from build123d import *

# Parameters (mm, degrees)
SKETCH1_R               = 6.25
BOSS_EXTRUDE1_DEPTH     = 15
SKETCH2_R               = 6.25
BOSS_EXTRUDE2_DEPTH     = 3
BOSS_EXTRUDE2_DRAFT     = -30
SKETCH3_R               = 6.25
BOSS_EXTRUDE3_DEPTH     = 51
SKETCH4_R               = 2.38125
BOSS_EXTRUDE4_DEPTH     = 44
SKETCH5_W               = 4
SKETCH5_H               = 14.941049413
CUT_EXTRUDE1_DEPTH      = 10
CUT_EXTRUDE2_DEPTH      = 114.720510346
CUT_EXTRUDE2_DEPTH_BACK = 114.720510346
SKETCH6_R               = 2


with BuildPart() as part:
    # Sketch1 → Boss-Extrude1 (new body)
    with BuildSketch(Plane.XY):
        Circle(SKETCH1_R)
    extrude(amount=BOSS_EXTRUDE1_DEPTH)


with BuildPart() as boss_extrude2_tool:
    # Sketch2 → Boss-Extrude2 (with draft: the straight prism first)
    with BuildSketch(Plane.XY.offset(15)):
        Circle(SKETCH2_R)
    extrude(amount=BOSS_EXTRUDE2_DEPTH)
    # Boss-Extrude2: the draft: its side faces are tilted about the plane it starts from
    boss_extrude2_sides = [boss_extrude2_tool.faces().sort_by_distance(p)[0] for p in [
        (-6.25, 0, 16.5),
    ]]
    draft(boss_extrude2_sides, Plane.XY.offset(15), BOSS_EXTRUDE2_DRAFT)


with BuildPart() as part_1:
    add(part.part)

    # Boss-Extrude2: add boss_extrude2_tool
    add(boss_extrude2_tool.part)

    # Sketch3 → Boss-Extrude3 (add)
    with BuildSketch(Plane.XY.offset(18)):
        Circle(SKETCH3_R)
    extrude(amount=BOSS_EXTRUDE3_DEPTH)

    # Sketch4 → Boss-Extrude4 (add)
    with BuildSketch(Plane.XY.offset(69)):
        Circle(SKETCH4_R)
    extrude(amount=BOSS_EXTRUDE4_DEPTH)

    # Sketch5 → Cut-Extrude1 (cut)
    with BuildSketch(Plane(origin=(0, 0, 0), x_dir=(-1, 0, 0), z_dir=(0, 0, -1))):
        with Locations((0, 0.333395318)):
            Rectangle(SKETCH5_W, SKETCH5_H)
    extrude(amount=-CUT_EXTRUDE1_DEPTH, mode=Mode.SUBTRACT)

    # Sketch6 → Cut-Extrude2 (cut, two sides: drawn at the far end of the back side and taken through both)
    with BuildSketch(Plane.ZY.offset(-2).offset(-CUT_EXTRUDE2_DEPTH_BACK)):
        with Locations(Location((5, 0, 0), (0, 0, 270))):
            Circle(SKETCH6_R)
    extrude(amount=CUT_EXTRUDE2_DEPTH + CUT_EXTRUDE2_DEPTH_BACK, mode=Mode.SUBTRACT)


solid = part_1.part
CAD build for the part. Positions are in the model's coordinates, mm. A direction names the side the tool comes from. Round coordinates to 2 decimals unless told otherwise and drop trailing zeros. Loops run counter-clockwise (first coordinate to the right, second up) from the corner with the lowest first, then second, coordinate; pieces in that order, holes last.
(1) Which spindle directions (+Z, -Z, +X, -X, +Y, -Y) get a long thin tool onto all of the face, cutting with end or side? Do faces 1 (the flat face through (-5, -4, 18)), 2 (the flat face through (0, 0, 113)), 3 (the flat face through (2, -0.1, 2.7)). Say none if no direction does.
(2) Two-plate mould, pull along Y, no slides. Class faces 4 (the flat face through (0, -3, 69)), 5 (the cylindrical face through (5.773, -2.394, 7.395)), 6 (the cylindrical face through (-4, 2, 5)): +Y half, -Y half, draft (parallel to the pull), parting line (faces both ways), or undercut.
(3) Drop flat-ended pins along their axis: pin 1 (8 mm diameter, centred on y = 0.5, z = 2.5, fed in from -X); pin 2 (1.5 mm diameter, centred on x = -1, y = -6, fed in from +Z); pin 3 (1 mm diameter, centred on x = 6, z = 45.5, fed in from -Y). Give the stop position or say it passes through.
(4) Cut at B-B (z = 5). Give the cut face in (x, y), plus the area to 3 significant figures.
(5) Cut at A-A (y = 0). Give the cut face in (x, z), plus the area to 3 significant figures.
(6) Wall check: line 1 along Z through (x, y) = (-2.75, -0.25); line 2 along Z through (x, y) = (-3.5, 2.75); line 3 along Y through (x, z) = (4.3, 5). Give the ranges that are in metal, low to high.
(7) Cut at C-C (x = 0). Give the cut face in (y, z), plus the area to 3 significant figures.
Findings below:
1. face 1: +Z
1. face 2: +Z, +X, -X, +Y, -Y
1. face 3: -Z, +Y, -Y
2. face 4: draft
2. face 5: parting line
2. face 6: undercut
3. pin 1: stops at x = -6.25
3. pin 2: stops at z = 69
3. pin 3: stops at y = -2.97
4. outline: (-5.92, -2) arc R6.25 ccw to (-2, -5.92) - (-2, -2) - close; (-5.92, 2) - (-2, 2) - (-2, 5.92) arc R6.25 ccw to start; (2, -5.92) arc R6.25 ccw to (5.92, -2) - (2, -2) - close; (2, 2) - (5.92, 2) arc R6.25 ccw to (2, 5.92) - close
4. area: 40.5 mm2
5. outline: (-7.98, 18) - (-6.25, 15) - (-6.25, 7) - (-2, 7) - (-2, 10) - (2, 10) - (2, 7) - (6.25, 7) - (6.25, 15) - (7.98, 18) - (6.25, 18) - (6.25, 69) - (2.38, 69) - (2.38, 113) - (-2.38, 113) - (-2.38, 69) - (-6.25, 69) - (-6.25, 18) - close; (-6.25, 0) - (-2, 0) - (-2, 3) - (-6.25, 3) - close; (2, 0) - (6.25, 0) - (6.25, 3) - (2, 3) - close
5. area: 1,000 mm2
6. line 1: z = 0 to 3.02, 6.98 to 69
6. line 2: z = 0 to 69
6. line 3: y = -4.54 to -2, 2 to 4.54
7. outline: (-7.98, 18) - (-6.25, 15) - (-6.25, 10) - (6.25, 10) - (6.25, 15) - (7.98, 18) - (6.25, 18) - (6.25, 69) - (2.38, 69) - (2.38, 113) - (-2.38, 113) - (-2.38, 69) - (-6.25, 69) - (-6.25, 18) - close
7. area: 952 mm2
